Geometry check sheet. Reference: the model listing, model coordinates, mm. Face numbers are marked on the shaded views. A direction names the side the tool comes from. Round coordinates to 2 decimals unless told otherwise and drop trailing zeros. Loops run counter-clockwise (first coordinate to the right, second up) from the corner with the lowest first, then second, coordinate; pieces in that order, holes last. Notation, with made-up numbers: M 66,65.5 L 95,65.5 A18 ccw 95,98.5 Z; hole C 16.5,74.25 d4. An arc over 180 degrees is marked long. Answer in a Markdown table with one row per item. Add a question column.
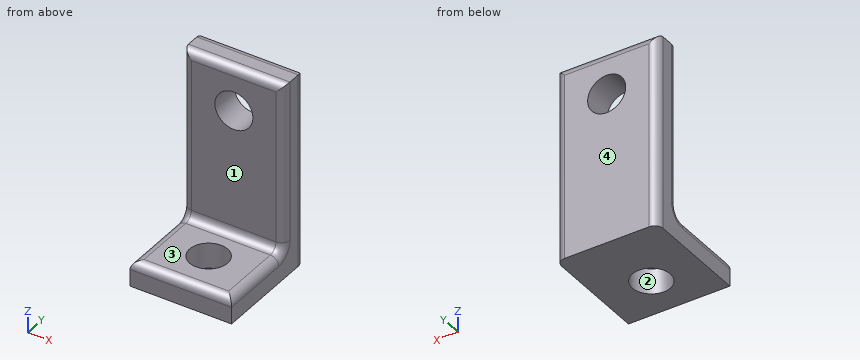
Autodesk Inventor part; units mm, degrees
ref_plane "YZ Plane" through (0, 0, 0) normal (1, 0, 0) x (0, 1, 0)
ref_plane "XZ Plane" through (0, 0, 0) normal (0, 1, 0) x (-1, 0, 0)
ref_plane "XY Plane" through (0, 0, 0) normal (0, 0, 1) x (1, 0, 0)
sketch "Sketch1" plane through (0, 0, 0) normal (0, 0, 1) x (1, 0, 0)
  circle A0 centre (0, 0) radius 2.25
  line L0 (-6, 4.5) -> (6, 4.5)
  line L1 (6, 4.5) -> (6, -5)
  line L2 (6, -5) -> (-6, -5)
  line L3 (-6, -5) -> (-6, 4.5)
  line L4 (-6, 4.5) -> (6, 4.5)
  line L5 (6, 4.5) -> (6, 8)
  line L6 (6, 8) -> (-6, 8)
  line L7 (-6, 8) -> (-6, 4.5)
  dimension "d0" = 4.5
  dimension "d1" = 5
  dimension "d2" = 6
  dimension "d3" = 6
  dimension "d4" = 4.5
  dimension "d5" = 3.5
extrude "Extrusion1" add sketch "Sketch1" along normal blind 3
sketch "Sketch2" plane through (0, 0, 3) normal (0, 0, 1) x (1, 0, 0)
  line L0 (-6, -5) -> (6, -5)
  line L1 (6, -5) -> (6, 8)
  line L2 (6, 8) -> (-6, 8)
  line L3 (-6, 8) -> (-6, -5)
  circle A0 centre (0, 0) radius 2.25
  line L4 (6, 8) -> (-6, 8)
  line L5 (-6, 8) -> (6, 8)
  line L6 (6, 8) -> (6, 4.5)
  line L7 (6, 4.5) -> (-6, 4.5)
  line L8 (-6, 4.5) -> (-6, 8)
  dimension "d8" = 3.5
extrude "Extrusion2" add sketch "Sketch2" along normal blind 20 contours L3 L2 L1 L7
sketch "Sketch3" plane through (-6, 8, 0) normal (0, 1, 0) x (1, 0, 0)
  point P0 (6, 0)
  point P1 (6.0288, -17.8643)
hole "Hole1" at (0.0288, 8, 17.8643) direction (0, -1, 0) diameter 4.5 depth 4 tip angle 118
fillet "Fillet1" radius 1 10 edges at (0, 4.5, 3) (0, 8, 23) (0, 4.5, 23) (0, -5, 3) (-6, -0.25, 3) (6, -0.25, 3) (6, 4.5, 13) (-6, 4.5, 13) (-6, 8, 11.5) (6, 8, 11.5)
properties part number "psu-bracket_3DPrint"
1) Cross-section at B-B, the plane x = -3.5. Record the boundary of the cut face in (y, z), plus the area to 3 significant figures.
2) Thickness scan on L1, parallel to Y at x = 0, z = 1.7; L2, parallel to Y at x = -3.5, z = 18.25; L3, parallel to Z at x = -4.5, y = 2.75. Record the ranges inside material, lowest first. Write a range as [from, to].
3) Draft check along X on the marked faces 1 and 2. Enter one of: +X half, -X half, draft (parallel to the pull), parting line (faces both ways), or undercut.
4) Cross-section at D-D, the plane x = -0.75. Record the boundary of the cut face in (y, z), plus the area to 3 significant figures.
5) Cross-section at A-A, the plane y = 0. Record the boundary of the cut face in (x, z), plus the area to 3 significant figures.
6) Cross-section at C-C, the plane z = 5. Record the boundary of the cut face in (x, y).
7) Go/stop test with a flat-tipped pin: pin 1 (2 mm diameter, centred on x = -4, y = 4, fed in from +Z). Record where the tip stops, or that it passes through.
8) Set-up check for the marked faces 3 and 4: record each of +Z, -Z, +X, -X, +Y, -Y from which the full face is reachable in a straight line by a thin tool's end or side.
Worked answers:
| question | item | result |
|---|---|---|
| 1 | outline | M -5,0 L 8,0 L 8,22 A1 ccw 7,23 L 5.5,23 A1 ccw 4.5,22 L 4.5,4 A1 cw 3.5,3 L -4,3 A1 ccw -5,2 Z |
| 1 | area | 109 mm2 |
| 2 | L1 | y = [-5, -2.25], [2.25, 8] |
| 2 | L2 | y = [4.5, 8] |
| 2 | L3 | z = [0, 3] |
| 3 | face 1 | draft |
| 3 | face 2 | undercut |
| 4 | outline | M -5,0 L -2.12,0 L -2.12,3 L -4,3 A1 ccw -5,2 Z; M 2.12,0 L 8,0 L 8,15.75 L 4.5,15.75 L 4.5,4 A1 cw 3.5,3 L 2.12,3 Z; M 4.5,19.98 L 8,19.98 L 8,22 A1 ccw 7,23 L 5.5,23 A1 ccw 4.5,22 Z |
| 4 | area | 81.1 mm2 |
| 5 | outline | M -6,0 L -2.25,0 L -2.25,3 L -5,3 A1 ccw -6,2 Z; M 2.25,0 L 6,0 L 6,2 A1 ccw 5,3 L 2.25,3 Z |
| 5 | area | 22.1 mm2 |
| 6 | outline | M -6,5.5 A1 ccw -5,4.5 L 5,4.5 A1 ccw 6,5.5 L 6,7 A1 ccw 5,8 L -5,8 A1 ccw -6,7 Z |
| 7 | pin 1 | stops at z = 22.87 |
| 8 | face 3 | +Z, +X, -X, -Y |
| 8 | face 4 | +Z, -Z, +X, -X, +Y |
